from build123d import *

# Parameters (mm, degrees)
SKETCH1_R           = 1.55
BOSS_EXTRUDE1_DEPTH = 4.5
SKETCH1_4_R         = 1.55
CUT_EXTRUDE1_DEPTH  = 2.5
BOSS_EXTRUDE2_DEPTH = 7.78
CUT_EXTRUDE2_REACH  = 68.276
CUT_EXTRUDE3_REACH  = 74.144
CUT_EXTRUDE4_REACH  = 74.144
CUT_EXTRUDE5_DEPTH  = 5


with BuildPart() as part:
    # Sketch1 → Boss-Extrude1 (new body)
    # profile 1 of 8: a face of its own
    with BuildSketch(Plane(origin=(0, 0, 0), x_dir=(0, 1, 0), z_dir=(0, 0, 1))):
        Polygon((-16.454482672, -28.5), (16.454482672, -28.5), (32.908965344, 0), (16.454482672, 28.5), (-16.454482672, 28.5), (-32.908965344, 0), align=None)
        Polygon((14.722431864, -25.5), (29.444863729, 0), (14.722431864, 25.5), (-14.722431864, 25.5), (-29.444863729, 0), (-14.722431864, -25.5), align=None, mode=Mode.SUBTRACT)
    # profile 2 of 8: a face of its own
    with BuildSketch(Plane(origin=(0, 0, 0), x_dir=(0, 1, 0), z_dir=(0, 0, 1))):
        Polygon((-14.722431864, -25.5), (14.722431864, -25.5), (29.444863729, 0), (14.722431864, 25.5), (-14.722431864, 25.5), (-29.444863729, 0), align=None)
        Polygon((-18.798769192, -3), (-17.066718385, 0), (-18.798769192, 3), (-22.262870808, 3), (-23.994921615, 0), (-22.262870808, -3), align=None, mode=Mode.SUBTRACT)
        Polygon((-8.533359192, -20.780211681), (-6.801308385, -17.780211681), (-8.533359192, -14.780211681), (-11.997460808, -14.780211681), (-13.729511615, -17.780211681), (-11.997460808, -20.780211681), align=None, mode=Mode.SUBTRACT)
        Polygon((11.997460808, -20.780211681), (13.729511615, -17.780211681), (11.997460808, -14.780211681), (8.533359192, -14.780211681), (6.801308385, -17.780211681), (8.533359192, -20.780211681), align=None, mode=Mode.SUBTRACT)
        Polygon((22.262870808, -3), (23.994921615, 0), (22.262870808, 3), (18.798769192, 3), (17.066718385, 0), (18.798769192, -3), align=None, mode=Mode.SUBTRACT)
        Polygon((11.997460808, 14.780211681), (13.729511615, 17.780211681), (11.997460808, 20.780211681), (8.533359192, 20.780211681), (6.801308385, 17.780211681), (8.533359192, 14.780211681), align=None, mode=Mode.SUBTRACT)
        Polygon((-8.533359192, 14.780211681), (-6.801308385, 17.780211681), (-8.533359192, 20.780211681), (-11.997460808, 20.780211681), (-13.729511615, 17.780211681), (-11.997460808, 14.780211681), align=None, mode=Mode.SUBTRACT)
    # profile 3 of 8: a face of its own
    with BuildSketch(Plane(origin=(0, 0, 0), x_dir=(0, 1, 0), z_dir=(0, 0, 1))):
        Polygon((8.533359192, -20.780211681), (11.997460808, -20.780211681), (13.729511615, -17.780211681), (11.997460808, -14.780211681), (8.533359192, -14.780211681), (6.801308385, -17.780211681), align=None)
        with Locations(Location((10.26541, -17.780211681, 0), (0, 0, 270))):
            Circle(SKETCH1_R, mode=Mode.SUBTRACT)
    # profile 4 of 8: a face of its own
    with BuildSketch(Plane(origin=(0, 0, 0), x_dir=(0, 1, 0), z_dir=(0, 0, 1))):
        Polygon((-11.997460808, -20.780211681), (-8.533359192, -20.780211681), (-6.801308385, -17.780211681), (-8.533359192, -14.780211681), (-11.997460808, -14.780211681), (-13.729511615, -17.780211681), align=None)
        with Locations(Location((-10.26541, -17.780211681, 0), (0, 0, 270))):
            Circle(SKETCH1_R, mode=Mode.SUBTRACT)
    # profile 5 of 8: a face of its own
    with BuildSketch(Plane(origin=(0, 0, 0), x_dir=(0, 1, 0), z_dir=(0, 0, 1))):
        Polygon((-22.262870808, -3), (-18.798769192, -3), (-17.066718385, 0), (-18.798769192, 3), (-22.262870808, 3), (-23.994921615, 0), align=None)
        with Locations(Location((-20.53082, 0, 0), (0, 0, 270))):
            Circle(SKETCH1_R, mode=Mode.SUBTRACT)
    # profile 6 of 8: a face of its own
    with BuildSketch(Plane(origin=(0, 0, 0), x_dir=(0, 1, 0), z_dir=(0, 0, 1))):
        Polygon((-11.997460808, 14.780211681), (-8.533359192, 14.780211681), (-6.801308385, 17.780211681), (-8.533359192, 20.780211681), (-11.997460808, 20.780211681), (-13.729511615, 17.780211681), align=None)
        with Locations(Location((-10.26541, 17.780211681, 0), (0, 0, 270))):
            Circle(SKETCH1_R, mode=Mode.SUBTRACT)
    # profile 7 of 8: a face of its own
    with BuildSketch(Plane(origin=(0, 0, 0), x_dir=(0, 1, 0), z_dir=(0, 0, 1))):
        Polygon((8.533359192, 14.780211681), (11.997460808, 14.780211681), (13.729511615, 17.780211681), (11.997460808, 20.780211681), (8.533359192, 20.780211681), (6.801308385, 17.780211681), align=None)
        with Locations(Location((10.26541, 17.780211681, 0), (0, 0, 270))):
            Circle(SKETCH1_R, mode=Mode.SUBTRACT)
    # profile 8 of 8: a face of its own
    with BuildSketch(Plane(origin=(0, 0, 0), x_dir=(0, 1, 0), z_dir=(0, 0, 1))):
        Polygon((18.798769192, -3), (22.262870808, -3), (23.994921615, 0), (22.262870808, 3), (18.798769192, 3), (17.066718385, 0), align=None)
        with Locations(Location((20.53082, 0, 0), (0, 0, 270))):
            Circle(SKETCH1_R, mode=Mode.SUBTRACT)
    extrude(amount=BOSS_EXTRUDE1_DEPTH)

    # Sketch1<4> → Cut-Extrude1 (cut)
    # profile 1 of 6: a face of its own
    with BuildSketch(Plane(origin=(0, 0, 0), x_dir=(0, 1, 0), z_dir=(0, 0, 1))):
        Polygon((-11.997460808, 14.780211681), (-8.533359192, 14.780211681), (-6.801308385, 17.780211681), (-8.533359192, 20.780211681), (-11.997460808, 20.780211681), (-13.729511615, 17.780211681), align=None)
        with Locations(Location((-10.26541, 17.780211681, 0), (0, 0, 270))):
            Circle(SKETCH1_4_R, mode=Mode.SUBTRACT)
    # profile 2 of 6: a face of its own
    with BuildSketch(Plane(origin=(0, 0, 0), x_dir=(0, 1, 0), z_dir=(0, 0, 1))):
        Polygon((-22.262870808, -3), (-18.798769192, -3), (-17.066718385, 0), (-18.798769192, 3), (-22.262870808, 3), (-23.994921615, 0), align=None)
        with Locations(Location((-20.53082, 0, 0), (0, 0, 270))):
            Circle(SKETCH1_4_R, mode=Mode.SUBTRACT)
    # profile 3 of 6: a face of its own
    with BuildSketch(Plane(origin=(0, 0, 0), x_dir=(0, 1, 0), z_dir=(0, 0, 1))):
        Polygon((-11.997460808, -20.780211681), (-8.533359192, -20.780211681), (-6.801308385, -17.780211681), (-8.533359192, -14.780211681), (-11.997460808, -14.780211681), (-13.729511615, -17.780211681), align=None)
        with Locations(Location((-10.26541, -17.780211681, 0), (0, 0, 270))):
            Circle(SKETCH1_4_R, mode=Mode.SUBTRACT)
    # profile 4 of 6: a face of its own
    with BuildSketch(Plane(origin=(0, 0, 0), x_dir=(0, 1, 0), z_dir=(0, 0, 1))):
        Polygon((8.533359192, -20.780211681), (11.997460808, -20.780211681), (13.729511615, -17.780211681), (11.997460808, -14.780211681), (8.533359192, -14.780211681), (6.801308385, -17.780211681), align=None)
        with Locations(Location((10.26541, -17.780211681, 0), (0, 0, 270))):
            Circle(SKETCH1_4_R, mode=Mode.SUBTRACT)
    # profile 5 of 6: a face of its own
    with BuildSketch(Plane(origin=(0, 0, 0), x_dir=(0, 1, 0), z_dir=(0, 0, 1))):
        Polygon((18.798769192, -3), (22.262870808, -3), (23.994921615, 0), (22.262870808, 3), (18.798769192, 3), (17.066718385, 0), align=None)
        with Locations(Location((20.53082, 0, 0), (0, 0, 270))):
            Circle(SKETCH1_4_R, mode=Mode.SUBTRACT)
    # profile 6 of 6: a face of its own
    with BuildSketch(Plane(origin=(0, 0, 0), x_dir=(0, 1, 0), z_dir=(0, 0, 1))):
        Polygon((8.533359192, 14.780211681), (11.997460808, 14.780211681), (13.729511615, 17.780211681), (11.997460808, 20.780211681), (8.533359192, 20.780211681), (6.801308385, 17.780211681), align=None)
        with Locations(Location((10.26541, 17.780211681, 0), (0, 0, 270))):
            Circle(SKETCH1_4_R, mode=Mode.SUBTRACT)
    extrude(amount=CUT_EXTRUDE1_DEPTH, mode=Mode.SUBTRACT)

    # Sketch1<5> → Boss-Extrude2 (add)
    with BuildSketch(Plane(origin=(0, 0, 0), x_dir=(0, 1, 0), z_dir=(0, 0, 1))):
        Polygon((-16.454482672, -28.5), (16.454482672, -28.5), (32.908965344, 0), (16.454482672, 28.5), (-16.454482672, 28.5), (-32.908965344, 0), align=None)
        Polygon((14.722431864, -25.5), (29.444863729, 0), (14.722431864, 25.5), (-14.722431864, 25.5), (-29.444863729, 0), (-14.722431864, -25.5), align=None, mode=Mode.SUBTRACT)
    extrude(amount=BOSS_EXTRUDE2_DEPTH)

    # Cut-Extrude2: up to this face of the body (flat: up to its plane)
    cut_extrude2_end = Plane(part.part.faces().sort_by_distance((28.5, 0, 3.89))[0])
    # Sketch2 → Cut-Extrude2 (cut, up to the picked face)
    with BuildSketch(Plane(origin=(-28.5, 0, 0), x_dir=(0, -1, 0), z_dir=(-1, 0, 0)), mode=Mode.PRIVATE) as cut_extrude2_sk1:
        with BuildLine():
            Line((-2.75, 10.78), (2.75, 10.78))
            ThreePointArc((2.75, 10.78), (5.75, 7.78), (2.75, 4.78))
            Line((2.75, 4.78), (-2.75, 4.78))
            ThreePointArc((-2.75, 4.78), (-5.75, 7.78), (-2.75, 10.78))
        make_face()
    cut_extrude2_tool1 = split(extrude(cut_extrude2_sk1.sketch, amount=-CUT_EXTRUDE2_REACH, mode=Mode.PRIVATE), bisect_by=cut_extrude2_end, keep=Keep.BOTH, mode=Mode.PRIVATE)
    add(cut_extrude2_tool1.solids().sort_by(Axis((-28.5, 0, 7.78), (1, 0, 0)))[0], mode=Mode.SUBTRACT)

    # Cut-Extrude3: up to this face of the body (flat: up to its plane)
    cut_extrude3_end = Plane(part.part.faces().sort_by_distance((14.25, 24.681724008, 3.89))[0])
    # Sketch3 → Cut-Extrude3 (cut, up to the picked face)
    with BuildSketch(Plane(origin=(-14.25, -24.681724008, 0), x_dir=(0.8660254037844387, -0.49999999999999983, 0), z_dir=(-0.49999999999999983, -0.8660254037844387, 0)), mode=Mode.PRIVATE) as cut_extrude3_sk1:
        with BuildLine():
            Line((-2.75, 10.78), (2.75, 10.78))
            ThreePointArc((2.75, 10.78), (5.75, 7.78), (2.75, 4.78))
            Line((2.75, 4.78), (-2.75, 4.78))
            ThreePointArc((-2.75, 4.78), (-5.75, 7.78), (-2.75, 10.78))
        make_face()
    cut_extrude3_tool1 = split(extrude(cut_extrude3_sk1.sketch, amount=-CUT_EXTRUDE3_REACH, mode=Mode.PRIVATE), bisect_by=cut_extrude3_end, keep=Keep.BOTH, mode=Mode.PRIVATE)
    add(cut_extrude3_tool1.solids().sort_by(Axis((-14.25, -24.681724, 7.78), (0.49999999999999983, 0.8660254037844387, 0)))[0], mode=Mode.SUBTRACT)

    # Cut-Extrude4: up to this face of the body (flat: up to its plane)
    cut_extrude4_end = Plane(part.part.faces().sort_by_distance((-14.25, 24.681724008, 3.89))[0])
    # Sketch4 → Cut-Extrude4 (cut, up to the picked face)
    with BuildSketch(Plane(origin=(14.25, -24.681724008, 0), x_dir=(0.8660254037844385, 0.5000000000000004, 0), z_dir=(0.5000000000000003, -0.8660254037844384, 0)), mode=Mode.PRIVATE) as cut_extrude4_sk1:
        with BuildLine():
            Line((-2.75, 10.78), (2.75, 10.78))
            ThreePointArc((2.75, 10.78), (5.75, 7.78), (2.75, 4.78))
            Line((2.75, 4.78), (-2.75, 4.78))
            ThreePointArc((-2.75, 4.78), (-5.75, 7.78), (-2.75, 10.78))
        make_face()
    cut_extrude4_tool1 = split(extrude(cut_extrude4_sk1.sketch, amount=-CUT_EXTRUDE4_REACH, mode=Mode.PRIVATE), bisect_by=cut_extrude4_end, keep=Keep.BOTH, mode=Mode.PRIVATE)
    add(cut_extrude4_tool1.solids().sort_by(Axis((14.25, -24.681724, 7.78), (-0.5000000000000003, 0.8660254037844384, 0)))[0], mode=Mode.SUBTRACT)

    # Sketch7 → Cut-Extrude5 (cut)
    with BuildSketch(Plane.XY.offset(7.78)):
        Polygon((-26.5, -6.75), (-26.5, -15.299782134), (-19.095671476, -19.5746732), (-19.595671476, -20.440698604), (-27.5, -15.877132403), (-27.5, -6.75), align=None)
        Polygon((-27.5, 6.75), (-26.5, 6.75), (-26.5, 15.299782134), (-19.095671476, 19.5746732), (-19.595671476, 20.440698604), (-27.5, 15.877132403), align=None)
        Polygon((-7.404328524, -26.3246732), (0, -30.599564267), (7.404328524, -26.3246732), (7.904328524, -27.190698604), (0, -31.754264805), (-7.904328524, -27.190698604), align=None)
        Polygon((19.095671476, -19.5746732), (26.5, -15.299782134), (26.5, -6.75), (27.5, -6.75), (27.5, -15.877132403), (19.595671476, -20.440698604), align=None)
        Polygon((26.5, 6.75), (26.5, 15.299782134), (19.095671476, 19.5746732), (19.595671476, 20.440698604), (27.5, 15.877132403), (27.5, 6.75), align=None)
        Polygon((7.404328524, 26.3246732), (0, 30.599564267), (-7.404328524, 26.3246732), (-7.904328524, 27.190698604), (0, 31.754264805), (7.904328524, 27.190698604), align=None)
    extrude(amount=-CUT_EXTRUDE5_DEPTH, mode=Mode.SUBTRACT)


solid = part.part
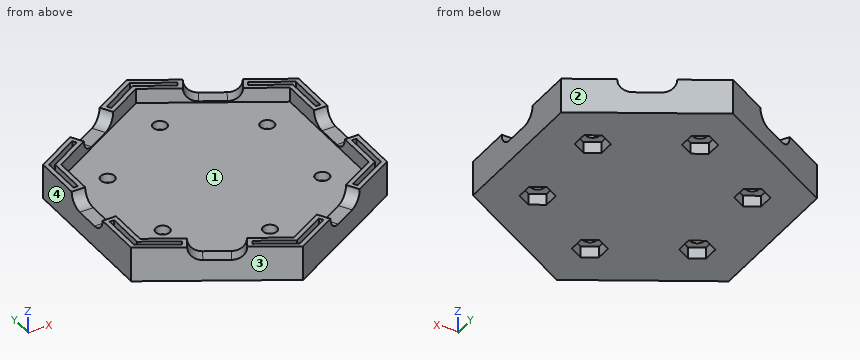
Can you work these out from the model? Positions are in its coordinate system, mm. Face numbers are marked on the shaded views. Give positions to 0.01 mm unless a question says otherwise; leave off trailing zeros. Loops run counter-clockwise (first coordinate to the right, second up) from the corner with the lowest first, then second, coordinate; pieces in that order, holes last. Notation, with made-up numbers: (71.5, 47) -> (86.5, 47) arc R21 ccw to (86.5, 56) -> close; hole circle Ø4 at (86, 8). An arc over 180 degrees is marked (long way). Use one line per item in the form item = value.
1) If we section it at B-B (z = 1.5): Count the separate pieces of the cut face and the enclosed holes in it, plus the area to 3 significant figures.
Answers:
separate_pieces = 1
enclosed_holes = 6
area = 2,630 mm²
2) We'd pull the mould along Y, two halves only. Please class the marked faces 1, 2, 3 and 4: released by +Y, released by -Y, zero draft, split by the parting line, or undercut.
Answers:
face_1 = undercut
face_2 = released by +Y
face_3 = released by -Y
face_4 = zero draft
3) If we section it at A-A (x = 4): Please give me the cut outline in (y, z).
Answers:
outline = (-30.6, 0) -> (30.6, 0) -> (30.6, 7.78) -> (29.44, 7.78) -> (29.44, 2.78) -> (28.29, 2.78) -> (28.29, 7.78) -> (27.14, 7.78) -> (27.14, 4.5) -> (-27.14, 4.5) -> (-27.14, 7.78) -> (-28.29, 7.78) -> (-28.29, 2.78) -> (-29.44, 2.78) -> (-29.44, 7.78) -> (-30.6, 7.78) -> close
4) Will these pins go through, and if not, where does the flat tip stop? pin 1 (2 mm diameter, centred on x = -14.5, y = 23, fed in from +Z); pin 2 (1.8 mm diameter, centred on x = 19, y = -10, fed in from -Z); pin 3 (4 mm diameter, centred on x = 17.78, y = 10.27, fed in from +Z); pin 4 (2.5 mm diameter, centred on x = 22, y = 16.5, fed in from +Z).
Answers:
pin_1 = 4.78
pin_2 = 2.5
pin_3 = 4.5
pin_4 = 7.78
5) I need wall thicknesses on line 1 along X through (y, z) = (11, 6.25); line 2 along Y through (x, z) = (0, 3.2); line 3 along X through (y, z) = (11, 2). Which ranges of each line are inside material? Lowest first, please.
Answers:
line_1 = -28.5 to -27.5, -26.5 to -25.5, 25.5 to 26.5, 27.5 to 28.5
line_2 = -32.91 to -31.75, -30.6 to -22.08, -18.98 to 18.98, 22.08 to 30.6, 31.75 to 32.91
line_3 = -28.5 to -20.78, -14.78 to 14.78, 20.78 to 28.5
